```python
from build123d import *

# Parameters (mm, degrees)
BOSS_EXTRUDE1_DEPTH = 20
SKETCH3_W           = 9
SKETCH3_H           = 7
BOSS_EXTRUDE2_DEPTH = 1


with BuildPart() as part:
    # Sketch1 → Boss-Extrude1 (new body)
    with BuildSketch(Plane.XY):
        Polygon((0, 0), (0, -7), (-9, -7), (-9, 0), (-7, 0), (-7, -5), (-2, -5), (-2, 0), align=None)
    extrude(amount=BOSS_EXTRUDE1_DEPTH)

    # Sketch3 → Boss-Extrude2 (add)
    with BuildSketch(Plane.XY.offset(20)):
        with Locations((-4.5, -3.5)):
            Rectangle(SKETCH3_W, SKETCH3_H)
    extrude(amount=BOSS_EXTRUDE2_DEPTH)


solid = part.part
```
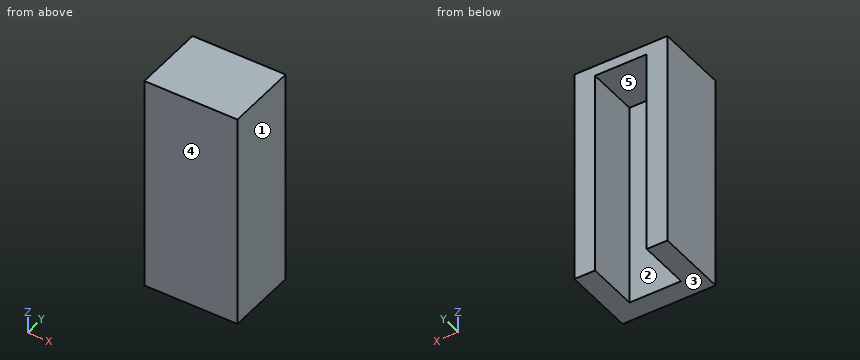
Work out the finished part from the listing and answer in its coordinate system (mm). Face numbers are marked on the shaded views. A direction names the side the tool comes from. Coordinates: 2 decimals unless noted, no trailing zeros. Order: outer loops, then holes, each group sorted by start corner. A loop starts at its lowest first (then second) coordinate and runs counter-clockwise, first axis right, second up. Notation, with made-up numbers: M 78,-4 L 132,-4 A12 cw 132,6 Z; hole C 25.25,12.25 d3. An arc over 180 degrees is marked long. Use CSV: the item, a comma, the result in double quotes.
1) For the marked faces 4 and 5, determine the directions among +Z, -Z, +X, -X, +Y, -Y from which every point of the face is accessible in a straight line to the end or side of a thin tool.
Worked out:
face 4,"+Z, -Z, +X, -X, -Y"
face 5,"-Z, +Y"
2) Section B-B on z = 6.5 is taken. Write down the section's boundary in (x, y).
Worked out:
outline,"M -9,-7 L 0,-7 L 0,0 L -2,0 L -2,-5 L -7,-5 L -7,0 L -9,0 Z"
3) Section A-A on y = -4.75 is taken. Write down the section's boundary in (x, z).
Worked out:
outline,"M -9,0 L -7,0 L -7,20 L -2,20 L -2,0 L 0,0 L 0,21 L -9,21 Z"
4) Consider line 1 (X direction, y = -0.5, z = 15); line 2 (Y direction, x = -4, z = 6.75); line 3 (Z direction, x = -6, y = -0.5). Determine where each line is inside the solid, lowest interval first. Write a range as [from, to].
Worked out:
line 1,"x = [-9, -7], [-2, 0]"
line 2,"y = [-7, -5]"
line 3,"z = [20, 21]"
5) Section C-C on x = -3.25 is taken. Write down the section's boundary in (y, z).
Worked out:
outline,"M -7,0 L -5,0 L -5,20 L 0,20 L 0,21 L -7,21 Z"
6) Determine the mould class of the marked faces 1, 2 and 3 for opening direction X: released by +X, released by -X, zero draft, split by the parting line, or undercut.
Worked out:
face 1,"released by +X"
face 2,"undercut"
face 3,"zero draft"
